Autodesk Inventor part; units mm, degrees
ref_plane "YZ Plane" through (0, 0, 0) normal (1, 0, 0) x (0, 1, 0)
ref_plane "XZ Plane" through (0, 0, 0) normal (0, 1, 0) x (-1, 0, 0)
ref_plane "XY Plane" through (0, 0, 0) normal (0, 0, 1) x (1, 0, 0)
sketch "スケッチ1" plane through (0, 0, 0) normal (1, 0, 0) x (0, 1, 0)
  arc A0 (8.4759, 50) -> (8.4759, -50) centre (234.0113, 0) ccw
  arc A1 (5.547, 50.6493) -> (5.547, -50.6493) centre (234.0113, 0) ccw
  line L0 (8.4759, 50) -> (5.547, 50.6493)
  line L1 (8.4759, -50) -> (5.547, -50.6493)
  line L2 (0, -70.909) -> (0, 70.909)
  point P0 (0, 0)
  point P1 (0, 0)
  dimension "d0" = 3
  dimension "d1" = 100
  dimension "d2" = 25
extrude "押し出し1" add sketch "スケッチ1" along normal blind 260
properties part number "element_4" material "CFRP"
Can you work these out from the model? Positions are in its coordinate system, mm. Round coordinates to 2 decimals unless told otherwise and drop trailing zeros. Write each loop counter-clockwise with the first axis right and the second up, starting at its lowest first coordinate (ties: lowest second). Pieces come first, ordered by that corner, then holes. Notation, with made-up numbers: (-24, 3) -> (-1, 3) arc R9 ccw to (-1, 11) -> close; hole circle Ø8 at (21, -36). An arc over 180 degrees is marked (long way). One line per question, with ' | ' between items. Start each with the question number.
1) Suppose I cut it at A-A on x = 83.5. Write out the boundary of the cut face in (y, z).
2) Suppose I cut it at B-B on z = -12. Write out the boundary of the cut face in (x, y).
3) If we mould it in two halves opening along Z, with no side actions, what happens to faces 1 (the cylindrical face through (128.2, 3, -0.7)), 2 (the cylindrical face through (128.2, 0, -0.7)), 3 (the flat face through (0, 1, 0))? For each: released by +Z, released by -Z, zero draft, split by the parting line, or undercut.
4) I need wall thicknesses on line 1 (Y direction, x = 44, z = -8.5); line 2 (Y direction, x = 218, z = 20.5). Which ranges of each line are inside material? Lowest first, please. Write a range as [from, to].
5) I'm going to push flat-ended pins straight in: P1, Ø4, axis at x = 104, z = 37, coming from the -Y side; P2, Ø2, axis at x = 204.5, z = 2, coming from the +Y side; P3, Ø2, axis at x = 179, y = 6, coming from the +Z side; P4, Ø12, axis at x = 226, z = 26.5, coming from the +Y side. Where does each tip first touch, or does it pass through?
Return value:
1) outline: (5.55, -50.65) -> (8.48, -50) arc R231.01 cw to (8.48, 50) -> (5.55, 50.65) arc R234.01 ccw to start
2) outline: (0, 0.31) -> (260, 0.31) -> (260, 3.31) -> (0, 3.31) -> close
3) face 1: undercut | face 2: split by the parting line | face 3: zero draft
4) line 1: y = [0.15, 3.16] | line 2: y = [0.9, 3.91]
5) P1: stops at y = 2.63 | P2: stops at y = 3.02 | P3: stops at z = 50.65 | P4: stops at y = 5.3
